from build123d import *

# Parameters (mm, degrees)
F1_DEPTH = 25


with BuildPart() as f1:
    # F0 (on Top) → F1 (new body)
    with BuildSketch(Plane.XY):
        with BuildLine():
            Line((-42, 0), (0, 0))
            Line((0, 0), (10, 0))
            Line((10, 0), (20, 0))
            Line((20, 0), (62, 0))
            Line((62, 0), (62, -20.750001))
            ThreePointArc((62, -20.750001), (62.585786, -22.164214), (64, -22.750001))
            Line((64, -22.750001), (77.499998, -22.750001))
            ThreePointArc((77.499998, -22.750001), (78.914212, -22.164214), (79.499998, -20.750001))
            Line((79.499998, -20.750001), (79.499998, -16.750001))
            ThreePointArc((79.499998, -16.750001), (78.914212, -15.335787), (77.499998, -14.750001))
            Line((77.499998, -14.750001), (70.499998, -14.750001))
            ThreePointArc((70.499998, -14.750001), (69.085785, -14.164214), (68.499998, -12.750001))
            Line((68.499998, -12.750001), (68.499998, 6))
            ThreePointArc((68.499998, 6), (67.914212, 7.414214), (66.499998, 8))
            Line((66.499998, 8), (20, 8))
            Line((20, 8), (0, 8))
            Line((0, 8), (-46.499998, 8))
            ThreePointArc((-46.499998, 8), (-47.914212, 7.414214), (-48.499998, 6))
            Line((-48.499998, 6), (-48.499998, -12.750001))
            ThreePointArc((-48.499998, -12.750001), (-49.085785, -14.164214), (-50.499998, -14.750001))
            Line((-50.499998, -14.750001), (-57.499998, -14.750001))
            ThreePointArc((-57.499998, -14.750001), (-58.914212, -15.335787), (-59.499998, -16.750001))
            Line((-59.499998, -16.750001), (-59.499998, -20.750001))
            ThreePointArc((-59.499998, -20.750001), (-58.914212, -22.164214), (-57.499998, -22.750001))
            Line((-57.499998, -22.750001), (-44, -22.750001))
            ThreePointArc((-44, -22.750001), (-42.585786, -22.164214), (-42, -20.750001))
            Line((-42, -20.750001), (-42, 0))
        make_face()
        with BuildLine():
            ThreePointArc((20, 8), (10, 18), (0, 8))
            Line((0, 8), (20, 8))
        make_face()
    extrude(amount=F1_DEPTH)


solid = f1.part
Source: CAD feature listing. Evaluate the final solid. Frame: model axes, mm. A direction names the side the tool comes from. Coordinates: 2 decimals unless noted, no trailing zeros. Loops run counter-clockwise (first coordinate to the right, second up) from the corner with the lowest first, then second, coordinate; pieces in that order, holes last. Notation, with made-up numbers: (35.25, 34.5) - (49.25, 34.5) arc R23 ccw to (49.25, 48.5) - close; hole circle Ø7 at (26.25, -17.5). An arc over 180 degrees is marked (long way). One line per item, written item: value. Start each with the question number.
1. Contact query for flat-ended pins moving along their axis: P1, Ø1.5, axis at x = 17, z = 4, coming from the +Y side; P2, Ø1, axis at x = 28, z = 7.5, coming from the +Y side; P3, Ø3, axis at y = 8.5, z = 5.5, coming from the -X side. Output: stop coordinate, or through.
2. Set-up query: faces 1 (the flat face through (-48.5, -3, 12)), 2 (the flat face through (10, 1, 25)), 3 (the flat face through (-42, -11, 12)), 4 (the flat face through (44, 8, 12)). Return all of +Z, -Z, +X, -X, +Y, -Y with unobstructed straight access to the full face (end or side cutting, diameter ignored); none if empty.
3. Section C-C (x = 10). Return the cut outline in (y, z).
4. Section B-B (z = 8.25). Return the cut outline in (x, y).
5. Ray query, L1, parallel to X at y = -2.5, z = 4.25; L2, parallel to Y at x = -23.5, z = 17; L3, parallel to X at y = 4.5, z = 9.25. Return the intervals inside material, ascending.
6. Section A-A (y = -2.5). Return the cut outline in (x, z), and give its area (3 significant figures).
7. Mould query, pull axis X, two halves, no side actions, for faces 5 (the flat face through (9, 0, 12)), 6 (the flat face through (-51, -22.75, 12)), 7 (the flat face through (62, -10, 12)), 8 (the flat face through (-59.5, -19, 12)). Classes: pulls with the +X half, pulls with the -X half, needs draft (parallel to the pull), parting line crosses it, or undercut.
8. Section D-D (y = 3.5). Return the cut outline in (x, z), and give its area (4 significant figures).
Verdict:
1. P1: stops at y = 15.81
1. P2: stops at y = 8
1. P3: stops at x = -48.23
2. face 1: +Z, -Z, -X, +Y
2. face 2: +Z, +X, -X, +Y, -Y
2. face 3: +Z, -Z, -Y
2. face 4: +Z, -Z, +X, +Y
3. outline: (0, 0) - (18, 0) - (18, 25) - (0, 25) - close
4. outline: (-59.5, -20.75) arc R2 ccw to (-57.5, -22.75) - (-44, -22.75) arc R2 ccw to (-42, -20.75) - (-42, 0) - (62, 0) - (62, -20.75) arc R2 ccw to (64, -22.75) - (77.5, -22.75) arc R2 ccw to (79.5, -20.75) - (79.5, -16.75) arc R2 ccw to (77.5, -14.75) - (70.5, -14.75) arc R2 cw to (68.5, -12.75) - (68.5, 6) arc R2 ccw to (66.5, 8) - (20, 8) arc R10 ccw to (0, 8) - (-46.5, 8) arc R2 ccw to (-48.5, 6) - (-48.5, -12.75) arc R2 cw to (-50.5, -14.75) - (-57.5, -14.75) arc R2 ccw to (-59.5, -16.75) - close
5. L1: x = -48.5 to -42, 62 to 68.5
5. L2: y = 0 to 8
5. L3: x = -48.5 to 68.5
6. outline: (-48.5, 0) - (-42, 0) - (-42, 25) - (-48.5, 25) - close; (62, 0) - (68.5, 0) - (68.5, 25) - (62, 25) - close
6. area: 325 mm2
7. face 5: undercut
7. face 6: needs draft
7. face 7: undercut
7. face 8: pulls with the -X half
8. outline: (-48.5, 0) - (68.5, 0) - (68.5, 25) - (-48.5, 25) - close
8. area: 2,925 mm2
